Here's the drawing with two shaded views (mm, measured from the low corner). I have some questions. Give positions to 0.01 mm unless a question says otherwise; leave off trailing zeros. Loops run counter-clockwise (first coordinate to the right, second up) from the corner with the lowest first, then second, coordinate; pieces in that order, holes last. Notation, with made-up numbers: M -29,39.5 L -21,39.5 A30 cw -21,66.5 Z; hole C -10.75,-35.75 d10. An arc over 180 degrees is marked long. Use a Markdown table: item, result. Add a question column.
1) Suppose I cut it at B-B on x = 7.5. List the corners of the cut face in (y, z) for me (3 decimals), and give its area (3 significant figures).
2) If I drill on line 1 along Z through (x, y) = (8.5, 3.5) (3 decimals); line 2 along X through (y, z) = (1.5, 9.5) (3 decimals); line 3 along X through (y, z) = (17.25, 3.75) (3 decimals), over which ranges is the centre line in solid material (lowest first)? Write a range as [from, to].
3) Will these pins go through, and if not, where does the flat tip stop? pin 1 Ø8 at (x, y) = (4.5, 4) entering from -Z (3 decimals); pin 2 Ø1 at (x, y) = (2, 10.5) entering from +Z (3 decimals).
4) Suppose I cut it at A-A on z = 18.5. List the corners of the cut face in (x, y) for me (3 decimals).
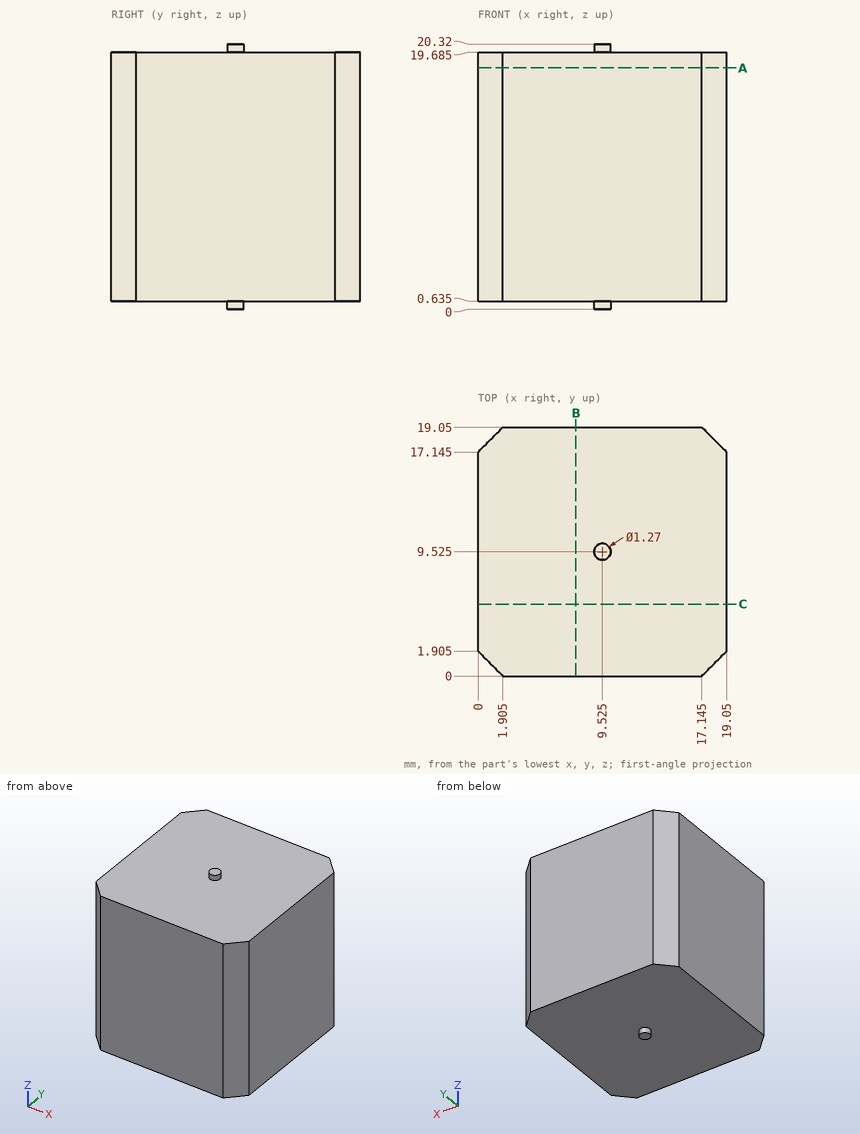
Answer block:
| question | item | result |
|---|---|---|
| 1 | outline | M 0,0.635 L 19.05,0.635 L 19.05,19.685 L 0,19.685 Z |
| 1 | area | 363 mm^2 |
| 2 | line 1 | z = [0.635, 19.685] |
| 2 | line 2 | x = [0.405, 18.645] |
| 2 | line 3 | x = [0.105, 18.945] |
| 3 | pin 1 | stops at z = 0.635 |
| 3 | pin 2 | stops at z = 19.685 |
| 4 | outline | M 0,1.905 L 1.905,0 L 17.145,0 L 19.05,1.905 L 19.05,17.145 L 17.145,19.05 L 1.905,19.05 L 0,17.145 Z |
